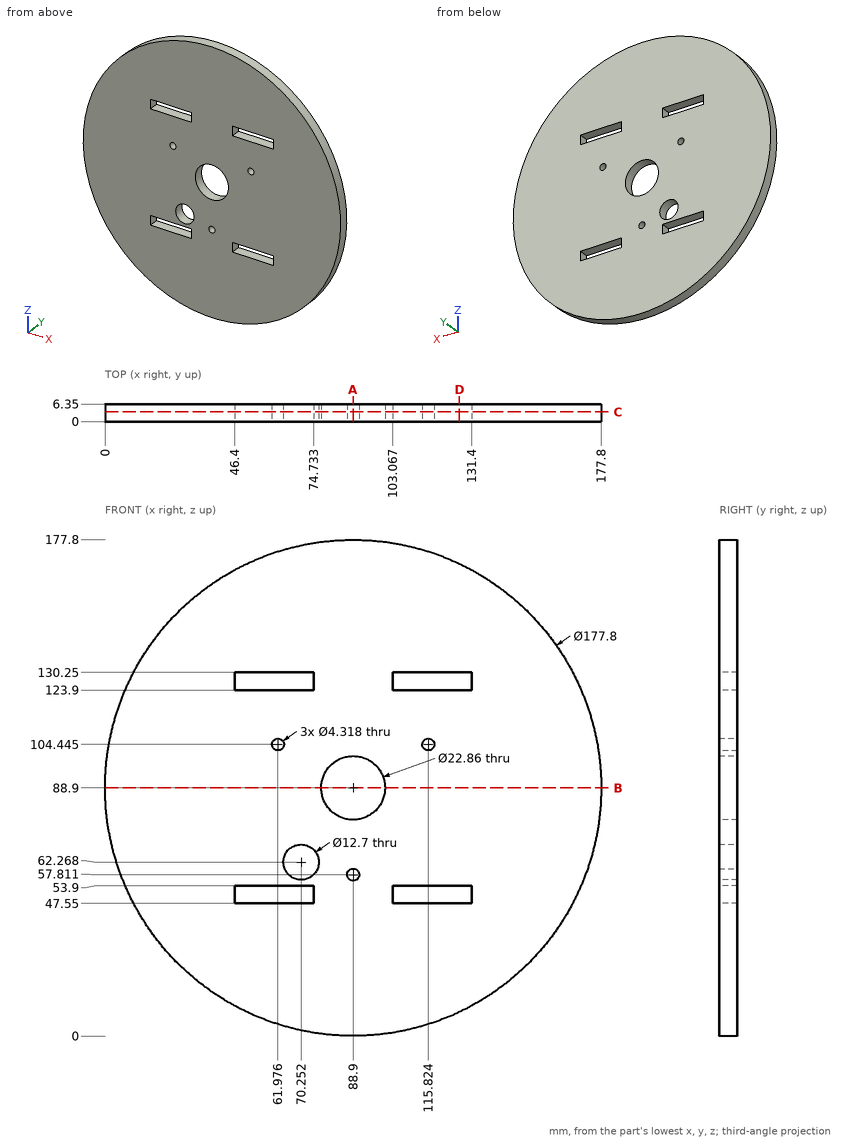
Here's the drawing with two shaded views (mm, measured from the low corner). I have some questions. Coordinates: 2 decimals unless noted, no trailing zeros. Order: outer loops, then holes, each group sorted by start corner. A loop starts at its lowest first (then second) coordinate and runs counter-clockwise, first axis right, second up. Notation, with made-up numbers: (86, 21) - (133, 21) arc R27 cw to (133, 41) - close; hole circle Ø11 at (40.25, -3). An arc over 180 degrees is marked (long way). Answer in a Markdown table with one row per item.
1. If I drill on line 1 along Z through (x, y) = (57, 2.5); line 2 along X through (y, z) = (5.5, 124) (1 decimal); line 3 along X through (y, z) = (4, 104), over which ranges is the centre line in solid material (lowest first)?
Reply:
| item | result |
|---|---|
| line 1 | z = 5.92 to 47.55, 53.9 to 123.9, 130.25 to 171.88 |
| line 2 | x = 7.2 to 46.4, 74.7 to 103.1, 131.4 to 170.6 |
| line 3 | x = 1.29 to 59.86, 64.09 to 113.71, 117.94 to 176.51 |
2. For pin 1 (3 mm diameter, centred on x = 20, y = 4.5, fed in from +Z); pin 2 (13.5 mm diameter, centred on x = 88.9, z = 88.9, fed in from -Y); pin 3 (1.5 mm diameter, centred on x = 106.5, y = 3, fed in from +Z); pin 4 (1 mm diameter, centred on y = 4.5, z = 155, fed in from +X), each with a flat end and sliding along its axis, tell me the tip position at first contact or that it passes through.
Reply:
| item | result |
|---|---|
| pin 1 | stops at z = 146.87 |
| pin 2 | passes through |
| pin 3 | stops at z = 176.19 |
| pin 4 | stops at x = 148.9 |
3. Suppose I cut it at D-D (x = 127). Please give me the cut outline in (y, z).
Reply:
| item | result |
|---|---|
| outline | (0, 8.58) - (6.35, 8.58) - (6.35, 47.55) - (0, 47.55) - close; (0, 53.9) - (6.35, 53.9) - (6.35, 123.9) - (0, 123.9) - close; (0, 130.25) - (6.35, 130.25) - (6.35, 169.22) - (0, 169.22) - close |
4. Suppose I cut it at B-B (z = 88.9). Please give me the cut outline in (x, y), and give its area (3 significant figures).
Reply:
| item | result |
|---|---|
| outline | (0, 0) - (77.47, 0) - (77.47, 6.35) - (0, 6.35) - close; (100.33, 0) - (177.8, 0) - (177.8, 6.35) - (100.33, 6.35) - close |
| area | 984 mm^2 |
5. Suppose I cut it at A-A (x = 88.9). Please give me the cut outline in (y, z).
Reply:
| item | result |
|---|---|
| outline | (0, 0) - (6.35, 0) - (6.35, 55.65) - (0, 55.65) - close; (0, 59.97) - (6.35, 59.97) - (6.35, 77.47) - (0, 77.47) - close; (0, 100.33) - (6.35, 100.33) - (6.35, 177.8) - (0, 177.8) - close |
6. Suppose I cut it at C-C (y = 3.5). Give the number of separate pieces and of enclosed holes in the cut face, and give its area (3 significant figures).
Reply:
| item | result |
|---|---|
| separate pieces | 1 |
| enclosed holes | 9 |
| area | 23,500 mm^2 |
